Read the model definition and answer for the solid it produces. Units are mm, in the model's axes. Round coordinates to 2 decimals unless told otherwise and drop trailing zeros. Write each loop counter-clockwise with the first axis right and the second up, starting at its lowest first coordinate (ties: lowest second). Pieces come first, ordered by that corner, then holes. Notation, with made-up numbers: (67.25, -24.5) - (76.25, -24.5) arc R17 ccw to (76.25, 7.5) - close; hole circle Ø7 at (3.25, 46). An arc over 180 degrees is marked (long way). Use one line per item in the form item = value. Start each with the question number.
1) The part is cut by section C-C, the plane x = -5. Give the vertices of the cut face in (y, z).
2) The part is cut by section A-A, the plane x = -35.5. Give the vertices of the cut face in (y, z), plus the area to 3 significant figures.
3) Each of these flat-tipped pins is pushed along its axis until it touches: pin 1 (1.1 mm diameter, centred on x = -39, z = 59, fed in from -Y); pin 2 (1 mm diameter, centred on x = -38.5, y = -2, fed in from +Z); pin 3 (5 mm diameter, centred on x = -54, z = 46.5, fed in from +Y). Where does it stop, or does it pass through?
4) The part is cut by section B-B, the plane z = 26. Give the vertices of the cut face in (x, y), plus the area to 3 significant figures.
5) Consider line 1 along Y through (x, z) = (-5, 41); line 2 along Z through (x, y) = (-35, -1.6). Determine where each line is inside the solid, lowest interval first. Write a range as from..to.
from build123d import *

# Parameters (mm, degrees)
F0_W     = 62.646739
F0_H     = 40.633425
F6_DEPTH = 1.33248
F1_R     = 2.621544
F2_R     = 1.49006
F2_R_2   = 1.453301
F2_R_3   = 1.619057
F2_R_4   = 1.451478
F3_DEPTH = 1.133365
F4_R     = 0.966379
F5_W     = 30.972634
F5_H     = 3.651396
F7_DEPTH = 0.337802


with BuildPart() as f6:
    # F0 (on Front) → F6 (new body)
    with BuildSketch(Plane.XZ):
        with Locations((-31.323369, 41.469335)):
            Rectangle(F0_W, F0_H)
    extrude(amount=F6_DEPTH)

    # F1
    f1_edges = [f6.edges().sort_by_distance(p)[0] for p in [
        (-62.646739, -0.66624, 21.152623),
        (-62.646739, -0.66624, 61.786048),
        (0, -0.66624, 61.786048),
        (0, -0.66624, 21.152623),
    ]]
    fillet(f1_edges, radius=F1_R)

    # F2 (on face) → F3 (join)
    with BuildSketch(Plane.XZ.offset(1.33248)):
        with Locations((-2.621544, 59.164504)):
            Circle(F2_R)
        with Locations((-60.025195, 23.774167)):
            Circle(F2_R_2)
        with Locations((-60.025195, 59.164504)):
            Circle(F2_R_3)
        with Locations((-2.621544, 23.774167)):
            Circle(F2_R_4)
    extrude(amount=F3_DEPTH)

    # F4
    f4_edges = [f6.edges().sort_by_distance(p)[0] for p in [
        (-4.073022, -2.465844, 23.774167),
        (-4.111604, -2.465844, 59.164504),
        (-61.478496, -2.465844, 23.774167),
        (-61.644252, -2.465844, 59.164504),
    ]]
    fillet(f4_edges, radius=F4_R)

    # F5 (on face) → F7 (join)
    with BuildSketch(Plane.XZ.offset(1.33248)):
        with Locations((-39.53187, 58.145337)):
            Rectangle(F5_W, F5_H)
    extrude(amount=F7_DEPTH)


solid = f6.part
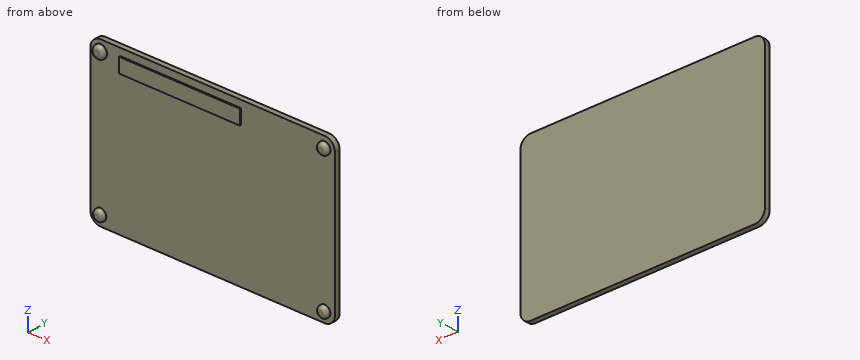
Geometry results:
q1.outline = (-1.33, 21.15) - (0, 21.15) - (0, 61.79) - (-1.33, 61.79) - close
q2.outline = (-1.67, 56.32) - (-1.33, 56.32) - (-1.33, 21.15) - (0, 21.15) - (0, 61.79) - (-1.33, 61.79) - (-1.33, 59.97) - (-1.67, 59.97) - close
q2.area = 55.4 mm2
q3.pin_1 = -1.67
q3.pin_2 = 59.97
q3.pin_3 = 0
q4.outline = (-62.65, -1.33) - (0, -1.33) - (0, 0) - (-62.65, 0) - close
q4.area = 83.5 mm2
q5.line_1 = -1.33..0
q5.line_2 = 56.32..59.97
